CAD build for the part. Positions are in the model's coordinates, mm. A direction names the side the tool comes from. Coordinates: 2 decimals unless noted, no trailing zeros. Loops run counter-clockwise (first coordinate to the right, second up) from the corner with the lowest first, then second, coordinate; pieces in that order, holes last. Notation, with made-up numbers: (19.25, -39.5) -> (55.25, -39.5) arc R15 ccw to (55.25, -15.5) -> close; hole circle Ø9 at (47.5, -12.5). An arc over 180 degrees is marked (long way). Write each question's results on one line, items separated by ' | '.
```python
from build123d import *

# Parameters (mm, degrees)
F0_W     = 7.85
F0_H     = 7.85
F1_DEPTH = 9.6
F2_R     = 2.45
F3_DEPTH = 1.9
F4_T     = -1.45
F5_SIZE  = 0.2


with BuildPart() as f1:
    # F0 (on Top) → F1 (new body)
    with BuildSketch(Plane.XY):
        Rectangle(F0_W, F0_H)
    extrude(amount=F1_DEPTH)

    # F2 (on face) → F3 (join)
    with BuildSketch(Plane.XY.offset(9.6)):
        Circle(F2_R)
    extrude(amount=F3_DEPTH)

    # F4
    f4_openings = [f1.faces().sort_by_distance(p)[0] for p in [
        (0, 0, 0),
    ]]
    offset(amount=F4_T, openings=f4_openings, kind=Kind.INTERSECTION)

    # F5
    f5_edges = [f1.edges().sort_by_distance(p)[0] for p in [
        (-2.45, 0, 11.5),
    ]]
    chamfer(f5_edges, length=F5_SIZE)


solid = f1.part
```
Q1. Drop flat-ended pins along their axis: pin 1 (1.5 mm diameter, centred on x = 0, y = 0.5, fed in from -Z); pin 2 (0.6 mm diameter, centred on x = 0, y = 0, fed in from -Z). Give the stop position or say it passes through.
Results are:
pin 1: z = 8.15 | pin 2: z = 10.05
Q2. Cut at C-C on y = 3.25. Write the cut outline in (x, z) (3 decimals).
Results are:
outline: (-3.925, 0) -> (3.925, 0) -> (3.925, 9.6) -> (-3.925, 9.6) -> close
Q3. Cut at B-B on z = 3.5. Write the cut outline in (x, y) (3 decimals).
Results are:
outline: (-3.925, -3.925) -> (3.925, -3.925) -> (3.925, 3.925) -> (-3.925, 3.925) -> close; hole (-2.475, -2.475) -> (2.475, -2.475) -> (2.475, 2.475) -> (-2.475, 2.475) -> close
Q4. Pull direction X, two halves, no side cores. Call faces 4 (the flat face through (-3.925, 0, 5)), 5 (the flat face through (0, 3.925, 5)), 6 (the flat face through (1, 1, 8.15)), 7 (the flat face through (0, 0, 10.05)): +X half, -X half, draft (parallel to the pull), parting line (faces both ways), or undercut.
Results are:
face 4: -X half | face 5: draft | face 6: undercut | face 7: undercut
Q5. Cut at A-A on x = 0. Write the cut outline in (y, z) (3 decimals), and give its area (3 significant figures).
Results are:
outline: (-3.925, 0) -> (-2.475, 0) -> (-2.475, 8.15) -> (-1, 8.15) -> (-1, 10.05) -> (1, 10.05) -> (1, 8.15) -> (2.475, 8.15) -> (2.475, 0) -> (3.925, 0) -> (3.925, 9.6) -> (2.45, 9.6) -> (2.45, 11.3) -> (2.25, 11.5) -> (-2.25, 11.5) -> (-2.45, 11.3) -> (-2.45, 9.6) -> (-3.925, 9.6) -> close | area: 40.5 mm^2
Q6. Which spindle directions (+Z, -Z, +X, -X, +Y, -Y) get a long thin tool onto all of the face, cutting with end or side? Do faces 1 (the flat face through (0, 0, 11.5)), 2 (the flat face through (2.475, 0, 4)), 3 (the flat face through (-2, 2, 9.6)). Say none if no direction does.
Results are:
face 1: +Z, +X, -X, +Y, -Y | face 2: -Z | face 3: +Z
Q7. Cut at D-D on z = 10.5. Write the cut outline in (x, y).
Results are:
outline: circle Ø4.9 at (0, 0)
Q8. Wall check: L1, parallel to Y at x = 0.75, z = 1.5 (3 decimals); L2, parallel to Y at x = 0, z = 9.1 (3 decimals). Give the ranges that are in metal, low to high. Write a range as from..to.
Results are:
L1: -3.925..-2.475, 2.475..3.925 | L2: -3.925..-1, 1..3.925
